from build123d import *

# Parameters (mm, degrees)
EXTRUDE1_DEPTH                                = 1.2
EXTRUDE_THIN1_DEPTH                           = 1.2
SKETCH9_R                                     = 2.7989
EXTRUDE3_DEPTH                                = 3.008
SKETCH11_OUTSIDE_W                            = 59.99
SKETCH11_OUTSIDE_H                            = 40.146
CUT_EXTRUDE2_DEPTH                            = 28.831479731
CSK_FOR_2_FLAT_HEAD_MACHINE_SCREW1_AT_2_COUNT = 2
CSK_FOR_2_FLAT_HEAD_MACHINE_SCREW1_AT_2_PITCH = 19.795
CSK_FOR_2_FLAT_HEAD_MACHINE_SCREW1_AT_3_COUNT = 2
CSK_FOR_2_FLAT_HEAD_MACHINE_SCREW1_AT_3_PITCH = 42.700459599
CSK_FOR_2_FLAT_HEAD_MACHINE_SCREW1_AT_4_COUNT = 2
CSK_FOR_2_FLAT_HEAD_MACHINE_SCREW1_AT_4_PITCH = 37.835


with BuildPart() as part:
    # Sketch2 → Extrude1 (new body)
    with BuildSketch(Plane.XY):
        with BuildLine():
            Line((22.1, -10.7046), (21.846, -10.7046))
            Line((21.846, -10.7046), (21.846, -12.6964))
            Line((21.846, -12.6964), (-21.846, -12.6964))
            Line((-21.846, -12.6964), (-21.846, -10.7046))
            Line((-21.846, -10.7046), (-22.1, -10.7046))
            Line((-22.1, -10.7046), (-23.54, -10.7046))
            Line((-23.54, -10.7046), (-23.54, 10.73))
            ThreePointArc((-23.54, 10.73), (-22.424076836, 13.424076836), (-19.73, 14.54))
            Line((-19.73, 14.54), (19.73, 14.54))
            ThreePointArc((19.73, 14.54), (22.424076836, 13.424076836), (23.54, 10.73))
            Line((23.54, 10.73), (23.54, -10.7046))
            Line((23.54, -10.7046), (22.1, -10.7046))
        make_face()
    extrude(amount=-EXTRUDE1_DEPTH)

    # Sketch3 → Extrude-Thin1 (add)
    with BuildSketch(Plane.XY):
        with BuildLine():
            Line((-19.814, -8.6726), (-19.814, -10.6644))
            Line((-19.814, -10.6644), (19.814, -10.6644))
            Line((19.814, -10.6644), (19.814, -8.6726))
            Line((19.814, -8.6726), (21.508, -8.6726))
            Line((21.508, -8.6726), (21.508, 10.73))
            ThreePointArc((21.508, 10.73), (20.987235857, 11.987235857), (19.73, 12.508))
            Line((19.73, 12.508), (-19.73, 12.508))
            ThreePointArc((-19.73, 12.508), (-20.987235857, 11.987235857), (-21.508, 10.73))
            Line((-21.508, 10.73), (-21.508, -8.6726))
            Line((-21.508, -8.6726), (-20.548, -8.6726))
            Line((-20.548, -8.6726), (-20.548, 10.73))
            ThreePointArc((-20.548, 10.73), (-20.308413347, 11.308413347), (-19.73, 11.548))
            Line((-19.73, 11.548), (19.73, 11.548))
            ThreePointArc((19.73, 11.548), (20.308413347, 11.308413347), (20.548, 10.73))
            Line((20.548, 10.73), (20.548, -7.7126))
            Line((20.548, -7.7126), (18.854, -7.7126))
            Line((18.854, -7.7126), (18.854, -9.7044))
            Line((18.854, -9.7044), (-18.854, -9.7044))
            Line((-18.854, -9.7044), (-18.854, -8.6726))
            Line((-18.854, -8.6726), (-19.814, -8.6726))
        make_face()
    extrude(amount=EXTRUDE_THIN1_DEPTH)

    # Sketch9 → Extrude3 (add)
    with BuildSketch(Plane.XY):
        with Locations(Location((18.9175, -9.8975, 0), (0, 0, 176.043941969))):
            Circle(SKETCH9_R)
        with Locations(Location((-18.9175, -9.8975, 0), (0, 0, 154.046840703))):
            Circle(SKETCH9_R)
        with Locations(Location((-18.9175, 9.8975, 0), (0, 0, 202.249746806))):
            Circle(SKETCH9_R)
        with Locations(Location((18.9175, 9.8975, 0), (0, 0, 143.864565))):
            Circle(SKETCH9_R)
    extrude(amount=EXTRUDE3_DEPTH)

    # Sketch11 outside → Cut-Extrude2 (cut, through all)
    with BuildSketch(Plane.XY):
        with Locations((0, 0.922)):
            Rectangle(SKETCH11_OUTSIDE_W, SKETCH11_OUTSIDE_H)
        with BuildLine():
            Line((-21.508, 10.73), (-21.508, -12.6964))
            Line((-21.508, -12.6964), (21.508, -12.6964))
            Line((21.508, -12.6964), (21.508, 10.73))
            ThreePointArc((21.508, 10.73), (20.987235857, 11.987235857), (19.73, 12.508))
            Line((19.73, 12.508), (-19.73, 12.508))
            ThreePointArc((-19.73, 12.508), (-20.987235857, 11.987235857), (-21.508, 10.73))
        make_face(mode=Mode.SUBTRACT)
    extrude(amount=CUT_EXTRUDE2_DEPTH, mode=Mode.SUBTRACT)

    # Sketch7 → CSK for #2 Flat Head Machine Screw1 (revolve, cut)
    with BuildSketch(Plane(origin=(18.9175, 9.8975, -1.2), x_dir=(0, 1, 0), z_dir=(1, 0, 0))):
        Polygon((0, 0), (0, 4.208), (1.2192, 4.208), (1.2192, 1.364335587), (2.1844, 0.254), (2.1844, 0), align=None)
    csk_for_2_flat_head_machine_screw1 = revolve(axis=Axis((18.9175, 9.8975, -7.55), (0, 0, 1)), mode=Mode.SUBTRACT)

    # CSK for #2 Flat Head Machine Screw1 at 2: CSK for #2 Flat Head Machine Screw1 ×2
    with Locations(*[(0, -i * CSK_FOR_2_FLAT_HEAD_MACHINE_SCREW1_AT_2_PITCH, 0) for i in range(1, CSK_FOR_2_FLAT_HEAD_MACHINE_SCREW1_AT_2_COUNT)]):
        add(csk_for_2_flat_head_machine_screw1, mode=Mode.SUBTRACT)

    # CSK for #2 Flat Head Machine Screw1 at 3: CSK for #2 Flat Head Machine Screw1 ×2
    with Locations(*[Vector(-0.8860560367488772, -0.46357814847215617, 0) * (i * CSK_FOR_2_FLAT_HEAD_MACHINE_SCREW1_AT_3_PITCH) for i in range(1, CSK_FOR_2_FLAT_HEAD_MACHINE_SCREW1_AT_3_COUNT)]):
        add(csk_for_2_flat_head_machine_screw1, mode=Mode.SUBTRACT)

    # CSK for #2 Flat Head Machine Screw1 at 4: CSK for #2 Flat Head Machine Screw1 ×2
    with Locations(*[(-i * CSK_FOR_2_FLAT_HEAD_MACHINE_SCREW1_AT_4_PITCH, 0, 0) for i in range(1, CSK_FOR_2_FLAT_HEAD_MACHINE_SCREW1_AT_4_COUNT)]):
        add(csk_for_2_flat_head_machine_screw1, mode=Mode.SUBTRACT)


solid = part.part
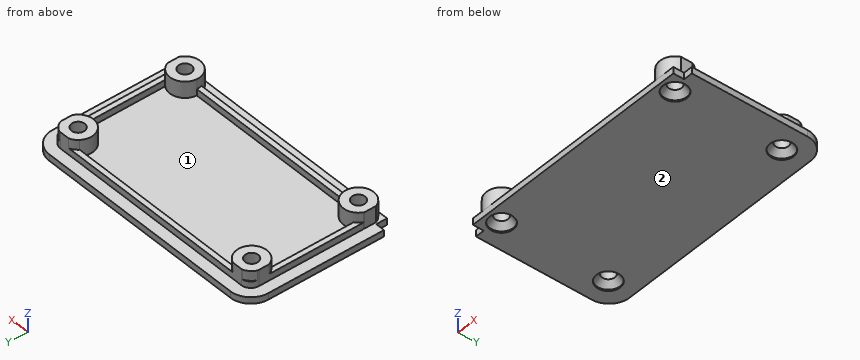
Can you work these out from the model? Positions are in its coordinate system, mm. Face numbers are marked on the shaded views. Give positions to 0.01 mm unless a question says otherwise; leave off trailing zeros. Loops run counter-clockwise (first coordinate to the right, second up) from the corner with the lowest first, then second, coordinate; pieces in that order, holes last. Notation, with made-up numbers: (1.5, 36) -> (23.5, 36) arc R29 ccw to (23.5, 68) -> close; hole circle Ø1 at (-31.5, 49). An arc over 180 degrees is marked (long way). Return JSON: item names as keys, results as strings.
Q1. For pin 1 Ø2.5 at (y, z) = (-10, 2) entering from +X; pin 2 Ø3 at (x, y) = (0, -5.5) entering from +Z; pin 3 Ø0.6 at (y, z) = (-9.5, 2) entering from -X, each with a flat end and sliding along its axis, tell me the tip position at first contact or that it passes through.
Checks:
{"pin 1": "stops at x = 21.51", "pin 2": "stops at z = 0", "pin 3": "stops at x = -21.51"}
Q2. I want a section at B-B, the plane x = 5.5. List the corners of the cut face in (y, z) for me.
Checks:
{"outline": "(-12.7, -1.2) -> (14.54, -1.2) -> (14.54, 0) -> (12.51, 0) -> (12.51, 1.2) -> (11.55, 1.2) -> (11.55, 0) -> (-9.7, 0) -> (-9.7, 1.2) -> (-10.66, 1.2) -> (-10.66, 0) -> (-12.7, 0) -> close"}
Q3. I want a section at A-A, the plane z = 0.65. List the corners of the cut face in (x, y) for me, then the cut area to 3 significant figures.
Checks:
{"outline": "(-21.51, -10.96) arc R2.8 ccw to (-16.23, -10.66) -> (16.23, -10.66) arc R2.8 ccw to (21.51, -10.96) -> (21.51, -8.84) arc R2.8 ccw to (21.43, -8.67) -> (21.51, -8.67) -> (21.51, 10.73) arc R1.78 ccw to (19.73, 12.51) -> (-19.73, 12.51) arc R1.78 ccw to (-21.51, 10.73) -> (-21.51, -8.67) -> (-21.43, -8.67) arc R2.8 ccw to (-21.51, -8.84) -> close; hole (-20.55, -7.62) arc R2.8 cw to (-16.13, -9.7) -> (16.13, -9.7) arc R2.8 cw to (20.55, -7.62) -> (20.55, 7.62) arc R2.8 cw to (16.66, 11.55) -> (-16.66, 11.55) arc R2.8 cw to (-20.55, 7.62) -> close; hole circle Ø2.44 at (-18.92, -9.9); hole circle Ø2.44 at (-18.92, 9.9); hole circle Ø2.44 at (18.92, -9.9); hole circle Ø2.44 at (18.92, 9.9)", "area": "174 mm2"}
Q4. I need wall thicknesses on probe 1 along Y at (x, z) = (19, 1.9); probe 2 along Y at (x, z) = (11, 0.85); probe 3 along X at (y, z) = (-10.75, 2.2). Which ranges of each line are inside material? Lowest first, please.
Checks:
{"probe 1": "y = -12.7 to -11.11, -8.68 to -7.1, 7.1 to 8.68, 11.11 to 12.51", "probe 2": "y = -10.66 to -9.7, 11.55 to 12.51", "probe 3": "x = -21.51 to -19.79, -18.05 to -16.25, 16.25 to 18.05, 19.79 to 21.51"}
Q5. We'd pull the mould along X, two halves only. Please class the marked faces 1 and 2: released by +X, released by -X, zero draft, split by the parting line, or undercut.
Checks:
{"face 1": "undercut", "face 2": "zero draft"}
Q6. I want a section at C-C, the plane y = -2.75. List the corners of the cut face in (x, z) for me, then the cut area to 3 significant figures.
Checks:
{"outline": "(-23.54, -1.2) -> (23.54, -1.2) -> (23.54, 0) -> (21.51, 0) -> (21.51, 1.2) -> (20.55, 1.2) -> (20.55, 0) -> (-20.55, 0) -> (-20.55, 1.2) -> (-21.51, 1.2) -> (-21.51, 0) -> (-23.54, 0) -> close", "area": "58.8 mm2"}
